Input: part model. Units: mm. Frame: model coordinates. Round coordinates to 2 decimals unless told otherwise and drop trailing zeros. Order: outer loops, then holes, each group sorted by start corner. A loop starts at its lowest first (then second) coordinate and runs counter-clockwise, first axis right, second up.
Item 1: Cut plane C-C on y = 21.5. Output: boundary loops of the cut face in (x, z).
Item 2: Cut plane A-A on z = -157.5. Output: boundary loops of the cut face in (x, y).
Item 3: First-contact query: pin 1 (1 mm diameter, centred on x = -396.5, y = 350.5, fed in from -Z). Flat tip, straight axial feed; report the tip coordinate or a pass-through.
Item 4: Cut plane B-B on x = 389. Output: boundary loops of the cut face in (y, z).
Item 5: Line query: L1, parallel to X at y = -414, z = -148; L2, parallel to Z at x = 746.5, y = -292.5. Output: solid intervals per line, ascending.
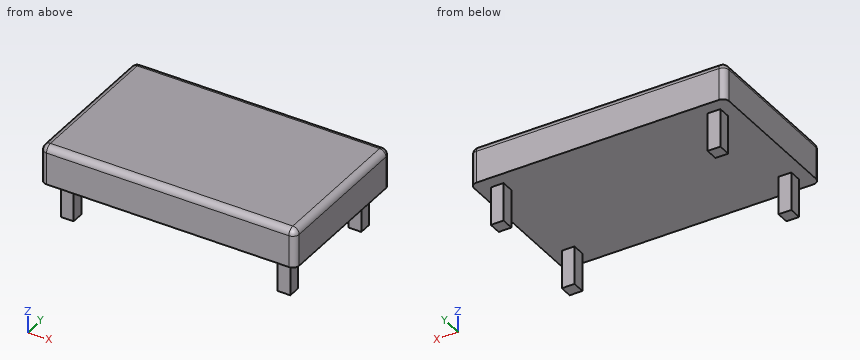
```python
from build123d import *

# Parameters (mm, degrees)
F0_W     = 2000
F0_H     = 1200
F1_DEPTH = 300
F2_R     = 50
F3_W     = 100
F3_H     = 100
F4_DEPTH = 300


with BuildPart() as f1:
    # F0 (on Top) → F1 (new body)
    with BuildSketch(Plane.XY):
        Rectangle(F0_W, F0_H)
    extrude(amount=F1_DEPTH)

    # F2
    f2_edges = [f1.edges().sort_by_distance(p)[0] for p in [
        (1000, 0, 300),
        (0, 600, 300),
        (-1000, 0, 300),
        (0, -600, 300),
        (-1000, -600, 150),
        (1000, -600, 150),
        (1000, 600, 150),
        (-1000, 600, 150),
    ]]
    fillet(f2_edges, radius=F2_R)

    # F3 (on face) → F4 (join)
    with BuildSketch(Plane(origin=(0, 0, 0), x_dir=(1, 0, 0), z_dir=(0, 0, -1))):
        with Locations((-850, 450)):
            Rectangle(F3_W, F3_H)
        with Locations((850, 450)):
            Rectangle(F3_W, F3_H)
        with Locations((-850, -450)):
            Rectangle(F3_W, F3_H)
        with Locations((850, -450)):
            Rectangle(F3_W, F3_H)
    extrude(amount=F4_DEPTH)


solid = f1.part
```
From the geometry:
1. outline: (-1000, 0) - (1000, 0) - (1000, 250) arc R50 ccw to (950, 300) - (-950, 300) arc R50 ccw to (-1000, 250) - close
2. outline: (-900, -500) - (-800, -500) - (-800, -400) - (-900, -400) - close; (-900, 400) - (-800, 400) - (-800, 500) - (-900, 500) - close; (800, -500) - (900, -500) - (900, -400) - (800, -400) - close; (800, 400) - (900, 400) - (900, 500) - (800, 500) - close
3. pin 1: stops at z = 0
4. outline: (-600, 0) - (600, 0) - (600, 250) arc R50 ccw to (550, 300) - (-550, 300) arc R50 ccw to (-600, 250) - close
5. L1: x = -900 to -800, 800 to 900
5. L2: z = 0 to 300
